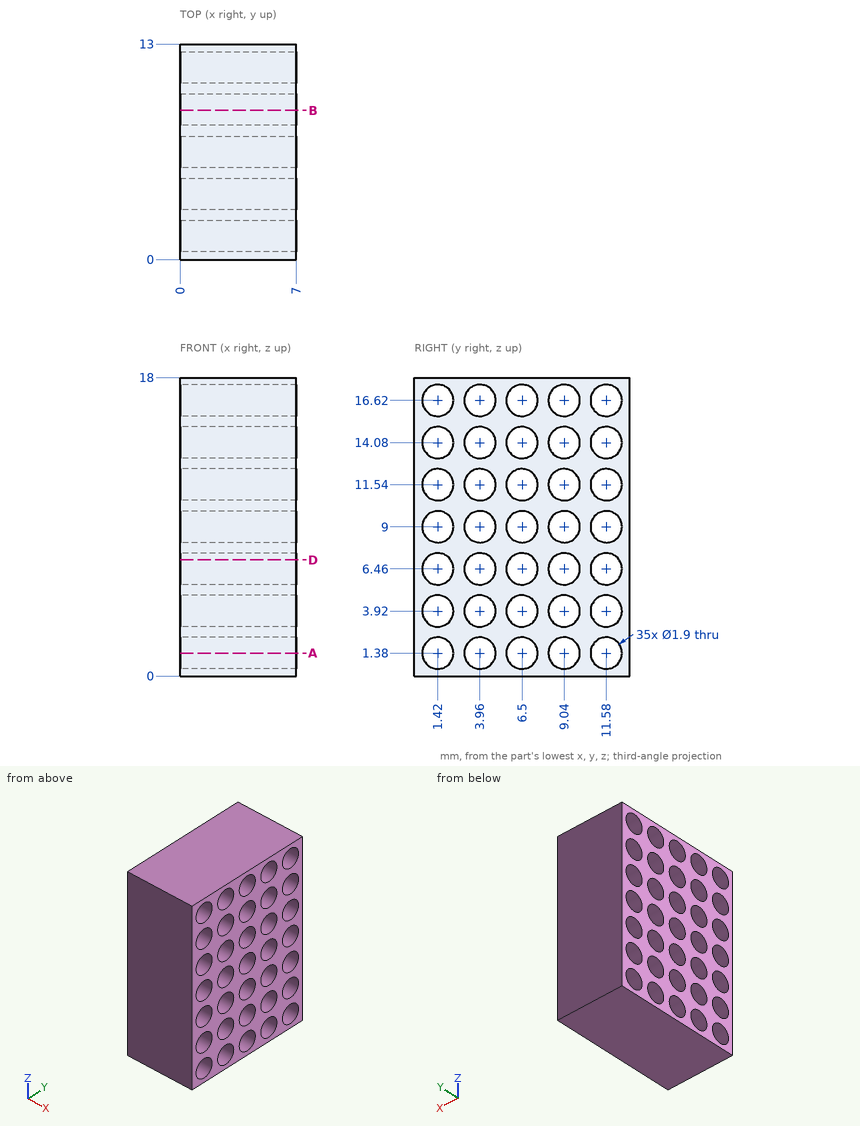
Verification items for this drawing (mm, ordinates from the low corner). Give positions to 0.01 mm unless a question says otherwise; leave off trailing zeros. Loops run counter-clockwise (first coordinate to the right, second up) from the corner with the lowest first, then second, coordinate; pieces in that order, holes last. Notation, with made-up numbers: M 14.5,30.25 L 56.5,30.25 A14 ccw 56.5,44.25 Z; hole C -19,33 d5. An arc over 180 degrees is marked long. Write item = value, one per line. Start each with the question number.
1. Section check A-A, the plane z = 1.38. Enter the section's corners in (x, y), plus the area to 3 significant figures.
2. Go/stop test with a flat-tipped pin: P1, Ø1.7, axis at y = 11.58, z = 3.92, coming from the +X side. Record where the tip stops, or that it passes through.
3. Section check B-B, the plane y = 9. Give the number of separate pieces and of enclosed holes in the cut face, plus the area to 3 significant figures.
4. Section check D-D, the plane z = 7. Enter the section's corners in (x, y), plus the area to 3 significant figures.
5. Thickness scan on probe 1 along Y at (x, z) = (1.5, 4.25); probe 2 along Y at (x, z) = (4.75, 6.25). Record the ranges inside material, lowest first.
Values follow:
q1.outline = M 0,0 L 7,0 L 7,0.47 L 0,0.47 Z; M 0,2.37 L 7,2.37 L 7,3.01 L 0,3.01 Z; M 0,4.91 L 7,4.91 L 7,5.55 L 0,5.55 Z; M 0,7.45 L 7,7.45 L 7,8.09 L 0,8.09 Z; M 0,9.99 L 7,9.99 L 7,10.63 L 0,10.63 Z; M 0,12.53 L 7,12.53 L 7,13 L 0,13 Z
q1.area = 24.5 mm^2
q2.P1 = through
q3.separate_pieces = 8
q3.enclosed_holes = 0
q3.area = 33.0 mm^2
q4.outline = M 0,0 L 7,0 L 7,0.64 L 0,0.64 Z; M 0,2.2 L 7,2.2 L 7,3.18 L 0,3.18 Z; M 0,4.74 L 7,4.74 L 7,5.72 L 0,5.72 Z; M 0,7.28 L 7,7.28 L 7,8.26 L 0,8.26 Z; M 0,9.82 L 7,9.82 L 7,10.8 L 0,10.8 Z; M 0,12.36 L 7,12.36 L 7,13 L 0,13 Z
q4.area = 36.3 mm^2
q5.probe_1 = 0 to 0.53, 2.31 to 3.07, 4.85 to 5.61, 7.39 to 8.15, 9.93 to 10.69, 12.47 to 13
q5.probe_2 = 0 to 0.49, 2.35 to 3.03, 4.89 to 5.57, 7.43 to 8.11, 9.97 to 10.65, 12.51 to 13
